The listing builds one solid part. Answer for the finished solid, in the listing's coordinates (mm). A direction names the side the tool comes from. Coordinates: 2 decimals unless noted, no trailing zeros. Order: outer loops, then holes, each group sorted by start corner. A loop starts at its lowest first (then second) coordinate and runs counter-clockwise, first axis right, second up. Notation, with made-up numbers: (-6, -7) -> (27, -7) arc R21 ccw to (27, 8) -> close; hole circle Ø10 at (28, 59.5). An arc over 180 degrees is marked (long way). Answer in a Markdown table with one row per item.
```python
from build123d import *

# Parameters (mm, degrees)
SKETCH1_R               = 2.5
BOSS_EXTRUDE1_DEPTH     = 7
CUT_EXTRUDE1_DEPTH      = 8.842193571
CUT_EXTRUDE1_DEPTH_BACK = 8.842193571
SKETCH2_R               = 0.6
SKETCH3_R               = 1.002734692
BOSS_EXTRUDE2_DEPTH     = 4.3
SKETCH4_R               = 2.5
BOSS_EXTRUDE3_DEPTH     = 1.6


with BuildPart() as part:
    # Sketch1 → Boss-Extrude1 (new body)
    with BuildSketch(Plane(origin=(0, 0, 0), x_dir=(1, 0, 0), z_dir=(0, 1, 0))):
        with Locations(Location((0, 0, 0), (0, 0, 270))):
            Circle(SKETCH1_R)
    extrude(amount=BOSS_EXTRUDE1_DEPTH)

    # Sketch2 → Cut-Extrude1 (cut, two sides: drawn at the far end of the back side and taken through both)
    with BuildSketch(Plane.XY.offset(-CUT_EXTRUDE1_DEPTH_BACK)):
        with Locations(Location((0, 3, 0), (0, 0, 90.000000021))):
            Circle(SKETCH2_R)
    extrude(amount=CUT_EXTRUDE1_DEPTH + CUT_EXTRUDE1_DEPTH_BACK, mode=Mode.SUBTRACT)

    # Sketch3 → Boss-Extrude2 (add)
    with BuildSketch(Plane.XZ):
        with Locations(Location((0, 0, 0), (0, 0, 90))):
            Circle(SKETCH3_R)
    extrude(amount=BOSS_EXTRUDE2_DEPTH)

    # Sketch4 → Boss-Extrude3 (add)
    with BuildSketch(Plane.XZ.offset(4.3)):
        with Locations(Location((0, 0, 0), (0, 0, 90))):
            Circle(SKETCH4_R)
    extrude(amount=-BOSS_EXTRUDE3_DEPTH)


solid = part.part
```
(1) A cutting plane is placed at C-C, the plane z = 0. Determine the outline of the cut face in (x, y), then the cut area to 3 significant figures.
Check values:
| item | result |
|---|---|
| outline | (-2.5, -4.3) -> (2.5, -4.3) -> (2.5, -2.7) -> (1, -2.7) -> (1, 0) -> (2.5, 0) -> (2.5, 7) -> (-2.5, 7) -> (-2.5, 0) -> (-1, 0) -> (-1, -2.7) -> (-2.5, -2.7) -> close; hole circle Ø1.2 at (0, 3) |
| area | 47.3 mm² |
(2) A cutting plane is placed at A-A, the plane x = 0. Determine the outline of the cut face in (y, z), then the cut area to 3 significant figures.
Check values:
| item | result |
|---|---|
| outline | (-4.3, -2.5) -> (-2.7, -2.5) -> (-2.7, -1) -> (0, -1) -> (0, -2.5) -> (2.4, -2.5) -> (2.4, 2.5) -> (0, 2.5) -> (0, 1) -> (-2.7, 1) -> (-2.7, 2.5) -> (-4.3, 2.5) -> close; (3.6, -2.5) -> (7, -2.5) -> (7, 2.5) -> (3.6, 2.5) -> close |
| area | 42.4 mm² |
(3) Which of the six approach directions +Z, -Z, +X, -X, +Y, -Y give full straight-line access (tool end or side, diameter ignored) to faces 4 (the cylindrical face through (0.61, -1.331, -0.796)), 5 (the cylindrical face through (0.751, 3.451, 2.385))?
Check values:
| item | result |
|---|---|
| face 4 | none |
| face 5 | +Y, -Y |
(4) A cutting plane is placed at B-B, the plane z = -1.25. Determine the outline of the cut face in (x, y), then the cut area to 3 significant figures.
Check values:
| item | result |
|---|---|
| outline | (-2.17, -4.3) -> (2.17, -4.3) -> (2.17, -2.7) -> (-2.17, -2.7) -> close; (-2.17, 0) -> (2.17, 0) -> (2.17, 7) -> (-2.17, 7) -> close; hole circle Ø1.2 at (0, 3) |
| area | 36.1 mm² |
(5) A cutting plane is placed at D-D, the plane y = 5.75. Determine the outline of the cut face in (x, z), then the cut area to 3 significant figures.
Check values:
| item | result |
|---|---|
| outline | circle Ø5 at (0, 0) |
| area | 19.6 mm² |
(6) Find the intervals of material crossed by line 1 along Y through (x, z) = (-0.65, -1.8); line 2 along Y through (x, z) = (-0.05, -1.45); line 3 along X through (y, z) = (3, -0.1), in increasing order. Write a range as from..to.
Check values:
| item | result |
|---|---|
| line 1 | -4.3..-2.7, 0..7 |
| line 2 | -4.3..-2.7, 0..2.4, 3.6..7 |
| line 3 | -2.5..-0.6, 0.6..2.5 |
(7) For a pull along Y with two mould halves and no side action, classify faces 1 (the flat face through (0, 7, 0)), 2 (the flat face through (1, -2.7, 1)), 3 (the cylindrical face through (2.44, -3.51, -0.54)) as released by +Y, released by -Y, zero draft, split by the parting line, or undercut.
Check values:
| item | result |
|---|---|
| face 1 | released by +Y |
| face 2 | undercut |
| face 3 | zero draft |
(8) Flat-ended cylindrical pins translate along their axes: pin 1 (1.5 mm diameter, centred on y = -1, z = 2, fed in from +X); pin 2 (1 mm diameter, centred on y = 1, z = 2, fed in from -X). Find the tip coordinate at first contact, or state that the pin passes through.
Check values:
| item | result |
|---|---|
| pin 1 | through |
| pin 2 | x = -2 |
